from build123d import *

# Parameters (mm, degrees)
F0_W     = 20
F0_H     = 127
F0_W_2   = 1310
F1_DEPTH = 4
F2_D     = 30
F3_W     = 20
F3_H     = 127
F4_DEPTH = 2
F5_SIZE  = 2


with BuildPart() as f1:
    # F0 (on Front) → F1 (new body)
    with BuildSketch(Plane.XZ):
        with Locations((-665, 0)):
            Rectangle(F0_W, F0_H)
        Rectangle(F0_W_2, F0_H)
        with Locations((665, 0)):
            Rectangle(F0_W, F0_H)
    extrude(amount=F1_DEPTH)

    # F2 (through all)
    with Locations(Plane(origin=(0, 0, 0), x_dir=(1, 0, 0), z_dir=(0, 1, 0))):
        with Locations((623.46, -13.81)):
            Hole(F2_D / 2)

    # F3 (on face) → F4 (join)
    with BuildSketch(Plane.XZ.offset(4)):
        with Locations((-665, 0)):
            Rectangle(F3_W, F3_H)
        with Locations((665, 0)):
            Rectangle(F3_W, F3_H)
    extrude(amount=F4_DEPTH)

    # F5
    f5_edges = [f1.edges().sort_by_distance(p)[0] for p in [
        (675, 0, 0),
        (-675, 0, 0),
    ]]
    chamfer(f5_edges, length=F5_SIZE)


solid = f1.part
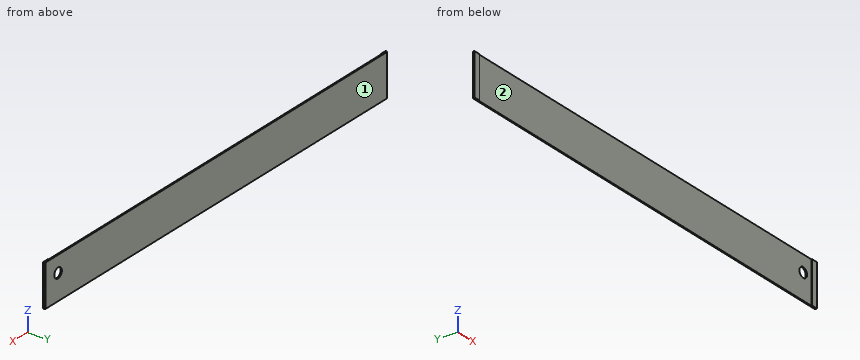
The listing builds one solid part. Answer for the finished solid, in the listing's coordinates (mm). Face numbers are marked on the shaded views. A direction names the side the tool comes from. Round coordinates to 2 decimals unless told otherwise and drop trailing zeros. Write each loop counter-clockwise with the first axis right and the second up, starting at its lowest first coordinate (ties: lowest second). Pieces come first, ordered by that corner, then holes. Notation, with made-up numbers: M 59,-34 L 118,-34 A32 ccw 118,2 Z; hole C -6.5,27 d6. An arc over 180 degrees is marked long. Write each question's results on one line, items separated by ' | '. Start each with the question number.
Item 1: A cutting plane is placed at C-C on z = -52. Write down the section's boundary in (x, y).
Item 2: A cutting plane is placed at D-D on x = -271.5. Write down the section's boundary in (y, z).
Item 3: A flat-ended cylindrical pin translates along its axis: pin 1 Ø5 at (x, z) = (-481, 12.5) entering from -Y. Find the tip coordinate at first contact, or state that the pin passes through.
Item 4: Straight lines are drawn through the part: L1, parallel to Z at x = 623.46, y = -2.45; L2, parallel to X at y = -2, z = 13; L3, parallel to X at y = -5, z = -9.5. For each, find the intervals that lie inside material, in ascending order. Write a range as [from, to].
Item 5: A cutting plane is placed at B-B on x = 623.46. Write down the section's boundary in (y, z).
Item 6: A cutting plane is placed at A-A on z = 13.81. Write down the section's boundary in (x, y).
Item 7: For the marked faces 1 and 2, determine the directions among +Z, -Z, +X, -X, +Y, -Y from which every point of the face is accessible in a straight line to the end or side of a thin tool.
Check sheet entries:
1) outline: M -675,-6 L -655,-6 L -655,-4 L 655,-4 L 655,-6 L 675,-6 L 675,-2 L 673,0 L -673,0 L -675,-2 Z
2) outline: M -4,-63.5 L 0,-63.5 L 0,63.5 L -4,63.5 Z
3) pin 1: y = -4
4) L1: [-63.5, -1.19], [28.81, 63.5] | L2: [-675, 608.48], [638.44, 675] | L3: [-675, -655], [655, 675]
5) outline: M -4,-63.5 L 0,-63.5 L 0,-1.19 L -4,-1.19 Z; M -4,28.81 L 0,28.81 L 0,63.5 L -4,63.5 Z
6) outline: M -675,-6 L -655,-6 L -655,-4 L 608.46,-4 L 608.46,0 L -673,0 L -675,-2 Z; M 638.46,-4 L 655,-4 L 655,-6 L 675,-6 L 675,-2 L 673,0 L 638.46,0 Z
7) face 1: +Z, -Z, +X, -X, +Y | face 2: +Z, -Z, -Y
